Can you work these out from the drawing? Everything is in mm from the part's minimum corner. A direction names the side the tool comes from. Give positions to 0.01 mm unless a question says otherwise; leave off trailing zeros. Order: outer loops, then holes, each group sorted by start corner. A loop starts at its lowest first (then second) coordinate and runs counter-clockwise, first axis right, second up. Notation, with made-up numbers: M -12.5,-40 L 33.5,-40 A4 cw 33.5,-33 Z; hole C 70.25,43.5 d9. An arc over 180 degrees is marked long. Answer as a JSON object with one key per item and string values.
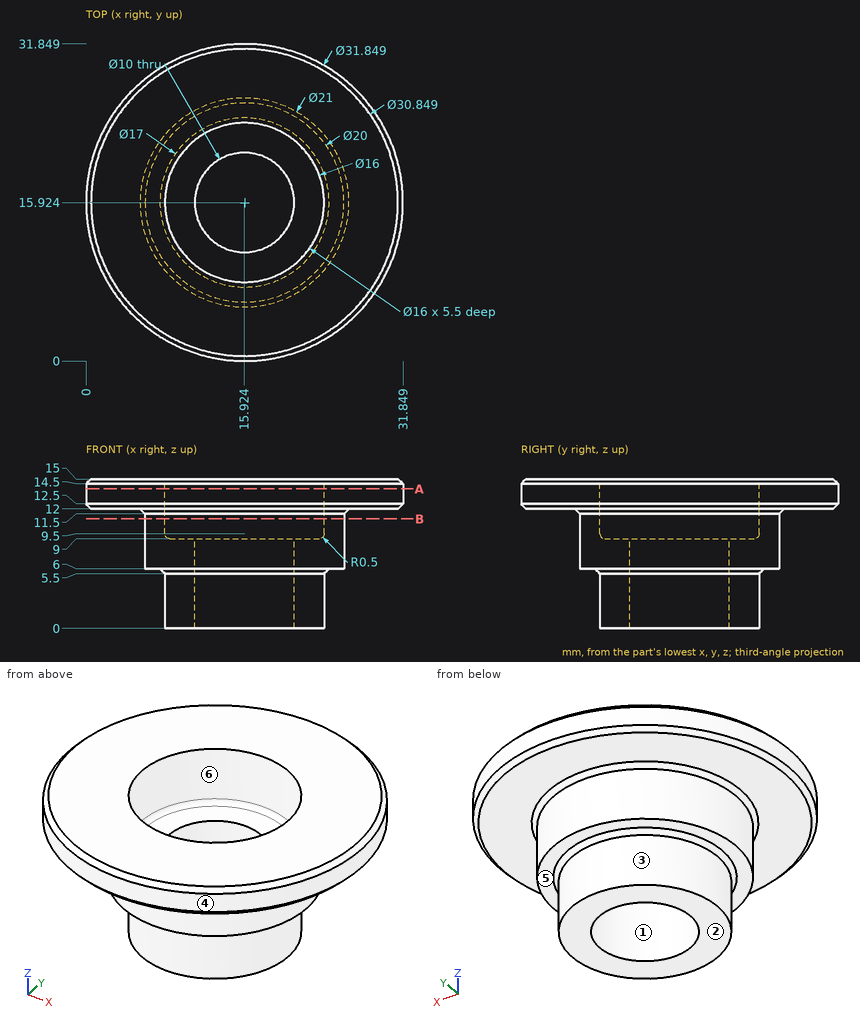
1) For the marked faces 4, 5 and 6, which set-ups out of +Z, -Z, +X, -X, +Y, -Y let a thin tool reach every point of the face, with its end or its side?
Results found:
{"face 4": "+Z, -Z", "face 5": "-Z", "face 6": "+Z"}
2) Thinking about a two-plate mould opening in X: for the marked faces 1, 2 and 3, which applies, pulls with the +X half, pulls with the -X half, needs draft (parallel to the pull), parting line crosses it, or undercut?
Results found:
{"face 1": "undercut", "face 2": "needs draft", "face 3": "parting line crosses it"}
3) I want a section at B-B on z = 11. Write out the boundary of the cut face in (x, y) (1 decimal), and give its area (3 significant figures).
Results found:
{"outline": "C 15.9,15.9 d20; hole C 15.9,15.9 d16", "area": "113 mm²"}
4) I want a section at A-A on z = 14. Write out the boundary of the cut face in (x, y) (1 decimal).
Results found:
{"outline": "C 15.9,15.9 d31.8; hole C 15.9,15.9 d16"}
5) I'm going to push flat-ended pins straight in: pin 1 Ø8 at (x, y) = (3.5, 12) entering from -Z; pin 2 Ø6 at (x, y) = (15.5, 13) entering from +Z; pin 3 Ø6 at (y, z) = (25, 7) entering from -X. Where does each tip first touch, or does it pass through?
Results found:
{"pin 1": "stops at z = 6", "pin 2": "stops at z = 9", "pin 3": "stops at x = 7.98"}
6) I need wall thicknesses on L1, parallel to Z at x = 27, y = 7; L2, parallel to Z at x = 9.5, y = 13; L3, parallel to Y at x = 13.5, z = 10.25 (1 decimal). Which ranges of each line are inside material? Lowest first, please.
Results found:
{"L1": "z = 12 to 15", "L2": "z = 0 to 9", "L3": "y = 6.2 to 8.3, 23.5 to 25.6"}
